Input: part model. Units: mm. Frame: model coordinates. A direction names the side the tool comes from. Give positions to 0.01 mm unless a question says otherwise; leave off trailing zeros. Loops run counter-clockwise (first coordinate to the right, second up) from the corner with the lowest first, then second, coordinate; pieces in that order, holes last.
Autodesk Inventor part; units mm, degrees
ref_plane "YZ Plane" through (0, 0, 0) normal (1, 0, 0) x (0, 1, 0)
ref_plane "XZ Plane" through (0, 0, 0) normal (0, 1, 0) x (-1, 0, 0)
ref_plane "XY Plane" through (0, 0, 0) normal (0, 0, 1) x (1, 0, 0)
sketch "Náčrt1" plane through (0, 0, 0) normal (0, 0, 1) x (1, 0, 0)
  point P0 (0, 0)
sketch "Náčrt2" plane through (0, 0, 0) normal (0, 0, 1) x (1, 0, 0)
  line L0 (17.2004, -10.497) -> (22.2004, -10.497)
  line L1 (-4.7996, 11.503) -> (-4.7996, 16.503)
  line L2 (-4.7996, 11.503) -> (17.2004, 11.503)
  line L3 (17.2004, -10.497) -> (17.2004, 11.503)
  line L4 (22.2004, -10.497) -> (22.2004, 11.503)
  line L5 (-4.7996, 16.503) -> (22.2004, 16.503)
  line L6 (22.2004, 11.503) -> (22.2004, 16.503)
  point P0 (0, 0)
  point P1 (15.2004, 9.503)
extrude "Vysunutí1" add sketch "Náčrt2" along normal blind 10
sketch "Náčrt3" plane through (0, 0, 10) normal (0, 0, 1) x (1, 0, 0)
  line L0 (17.2004, 11.503) -> (17.2004, -10.497)
  line L1 (22.2004, -10.497) -> (22.2004, 16.503)
  line L2 (22.2004, 16.503) -> (-4.7996, 16.503)
  line L3 (22.2004, 6.4599) -> (12.2431, 16.503)
  line L4 (12.2431, 16.503) -> (19.3444, 23.5436)
  line L5 (19.3444, 23.5436) -> (29.3017, 13.5006)
  line L6 (29.3017, 13.5006) -> (22.2004, 6.4599)
  point P0 (0, 0)
extrude "Vysunutí2" add sketch "Náčrt3" against normal blind 10 contours L1 L2 L4 L5 L6
sketch "Náčrt4" plane through (29.3017, 13.5006, 10) normal (0.7101, 0.7041, 0) x (0, 0, -1)
  point P0 (10, 11.0432)
sketch "Náčrt5" plane through (29.3017, 13.5006, 10) normal (0.7101, 0.7041, 0) x (0, 0, -1)
  line L0 (10, 0) -> (0, 0)
  line L1 (10, 22.5911) -> (10, 7.1016)
  line L2 (0, 14.1425) -> (10, 14.1425)
  line L3 (10, 7.1016) -> (10, -8.5213)
  line L4 (10, 7.1016) -> (0, 7.1016)
  circle A0 centre (5, 7.1016) radius 5
  point P0 (10, 11.0432)
extrude "Vysunutí3" add sketch "Náčrt5" along normal blind 50
sketch "Náčrt6" plane through (0, 0, 10) normal (0, 0, 1) x (1, 0, 0)
  line L0 (17.2004, 11.503) -> (17.2004, -10.497)
  line L1 (17.2004, -10.497) -> (17.2004, 4.503)
  line L2 (17.2004, 4.503) -> (15.2004, 4.503)
  line L3 (15.2004, 4.503) -> (15.2004, -10.497)
  line L4 (15.2004, -10.497) -> (17.2004, -10.497)
  line L5 (-4.7996, 11.503) -> (17.2004, 11.503)
  line L6 (-4.7996, 11.503) -> (-4.7996, 9.503)
  line L7 (-4.7996, 9.503) -> (10.2004, 9.503)
  line L8 (10.2004, 9.503) -> (10.2004, 11.503)
  line L9 (10.2004, 11.503) -> (-4.7996, 11.503)
  point P0 (0, 0)
extrude "Vysunutí4" add sketch "Náčrt6" against normal blind 10
properties part number "Součást3"
(1) Cut plane C-C (y = -4). Return the cut outline in (x, z), and give its area (3 significant figures).
Values follow:
outline: (15.2, 0) - (22.2, 0) - (22.2, 10) - (15.2, 10) - close
area: 70.0 mm2
(2) Pin query (flat end, axial travel): pin 1 Ø4 at (y, z) = (30, 4) entering from -X; pin 2 Ø1.6 at (y, z) = (10.5, 6) entering from +X; pin 3 Ø2 at (x, z) = (14, 7.5) entering from -Y. Return the tip coordinate at first contact, or that it passes through.
Values follow:
pin 1: stops at x = 26.83
pin 2: stops at x = 27.08
pin 3: stops at y = 11.5
(3) Ray query, probe 1 along Y at (x, z) = (-1.5, 5.25); probe 2 along X at (y, z) = (4, 6); probe 3 along Y at (x, z) = (21, 2.25). Return the intervals inside material, ascending.
Values follow:
probe 1: y = 9.5 to 16.5
probe 2: x = 15.2 to 22.2
probe 3: y = -10.5 to 21.87
(4) Cut plane A-A (z = 3). Return the cut outline in (x, y), and give its area (3 significant figures).
Values follow:
outline: (-4.8, 9.5) - (10.2, 9.5) - (10.2, 11.5) - (17.2, 11.5) - (17.2, 4.5) - (15.2, 4.5) - (15.2, -10.5) - (22.2, -10.5) - (22.2, 6.46) - (29.3, 13.5) - (27.53, 15.29) - (63.03, 50.49) - (56.58, 57) - (21.08, 21.8) - (19.34, 23.54) - (12.24, 16.5) - (-4.8, 16.5) - close
area: 855 mm2
(5) Reachability of faces 4 (the flat face through (22.2, -2, 5)), 5 (the flat face through (17.2, 8, 5)), 6 (the flat face through (15.2, -3, 5)) from +Z, -Z, +X, -X, +Y, -Y: full face, straight path, thin tool, end or side. Return the list, or none.
Values follow:
face 4: +Z, -Z, +X, -Y
face 5: +Z, -Z
face 6: +Z, -Z, -X, -Y
(6) Cut plane B-B (x = 9). Return the cut outline in (y, z).
Values follow:
outline: (9.5, 0) - (16.5, 0) - (16.5, 10) - (9.5, 10) - close
(7) Mould query, pull axis X, two halves, no side actions, for faces 1 (the flat face through (20.136, 22.745, 5.07)), 2 (the flat face through (59.757, 53.798, 5.07)), 3 (the flat face through (16, 4.503, 5)). Classes: +X half, -X half, draft (parallel to the pull), parting line (faces both ways), or undercut.
Values follow:
face 1: undercut
face 2: +X half
face 3: draft
(8) Cut plane D-D (z = 6.5). Return the cut outline in (x, y).
Values follow:
outline: (-4.8, 9.5) - (10.2, 9.5) - (10.2, 11.5) - (17.2, 11.5) - (17.2, 4.5) - (15.2, 4.5) - (15.2, -10.5) - (22.2, -10.5) - (22.2, 6.46) - (29.3, 13.5) - (27.66, 15.16) - (63.16, 50.36) - (56.45, 57.14) - (20.94, 21.93) - (19.34, 23.54) - (12.24, 16.5) - (-4.8, 16.5) - close
